```python
from build123d import *

# Parameters (mm, degrees)
F1_DEPTH = 50.8
F3_DEPTH = 12.7


with BuildPart() as f1:
    # F0 (on Top) → F1 (new body)
    with BuildSketch(Plane.XY):
        Polygon((0, 3.666174), (-3.175, 1.833087), (-3.175, -1.833087), (0, -3.666174), (3.175, -1.833087), (3.175, 1.833087), align=None)
    extrude(amount=F1_DEPTH)

    # F2 (on Front) → F3 (cut, symmetric)
    with BuildSketch(Plane.XZ):
        Polygon((-6.354235, 54.107219), (-6.183569, 46.427269), (5.677683, 50.864574), (5.677683, 54.107219), align=None)
    extrude(amount=F3_DEPTH, both=True, mode=Mode.SUBTRACT)


solid = f1.part
```
Here's how the part is built. I have some questions about the finished solid (model axes, mm). Round coordinates to 2 decimals unless told otherwise and drop trailing zeros. Order: outer loops, then holes, each group sorted by start corner. A loop starts at its lowest first (then second) coordinate and runs counter-clockwise, first axis right, second up. Notation, with made-up numbers: M -36,1.5 L -17,1.5 A33 ccw -17,36.5 Z; hole C 48.25,-18.5 d5. An arc over 180 degrees is marked long. Answer in a Markdown table with one row per item.
Item 1: I'm going to push a flat-ended pin straight in: pin 1 (4 mm diameter, centred on y = 2.5, z = 44, fed in from +X) (3 decimals). Where does the tip first touch, or does it pass through?
A:
| item | result |
|---|---|
| pin 1 | stops at x = 3.175 |
Item 2: Imagine slicing it at A-A, the plane z = 30.5. Write out the boundary of the cut face in (x, y) (3 decimals).
A:
| item | result |
|---|---|
| outline | M -3.175,-1.833 L 0,-3.666 L 3.175,-1.833 L 3.175,1.833 L 0,3.666 L -3.175,1.833 Z |
Item 3: If I drill on L1, parallel to Z at x = -1.25, y = -1.25; L2, parallel to X at y = -2, z = 22.5; L3, parallel to Y at x = 1.75, z = 36.5, over which ranges is the centre line in solid material (lowest first)? Write a range as from..to.
A:
| item | result |
|---|---|
| L1 | z = 0..48.27 |
| L2 | x = -2.89..2.89 |
| L3 | y = -2.66..2.66 |
Item 4: Imagine slicing it at C-C, the plane x = 2.25. Write out the boundary of the cut face in (y, z), and give its area (3 significant figures).
A:
| item | result |
|---|---|
| outline | M -2.37,0 L 2.37,0 L 2.37,49.58 L -2.37,49.58 Z |
| area | 235 mm2 |
Item 5: Imagine slicing it at B-B, the plane y = 0.5. Write out the boundary of the cut face in (x, z) (3 decimals), and give its area (3 significant figures).
A:
| item | result |
|---|---|
| outline | M -3.175,0 L 3.175,0 L 3.175,49.928 L -3.175,47.553 Z |
| area | 310 mm2 |
